Read the model definition and answer for the solid it produces. Units are mm, in the model's axes. A direction names the side the tool comes from. Coordinates: 2 decimals unless noted, no trailing zeros. Loops run counter-clockwise (first coordinate to the right, second up) from the corner with the lowest first, then second, coordinate; pieces in that order, holes last.
Q1. Straight lines are drawn through the part: line 1 (Y direction, x = 0, z = 95.7); line 2 (Z direction, x = 158, y = 115); line 3 (Y direction, x = 0, z = -96.3). For each, find the intervals that lie inside material, in ascending order.
Q2. Flat-ended cylindrical pins translate along their axes: P1, Ø2.5, axis at y = 77, z = 96.5, coming from the -X side (3 decimals); P2, Ø7, axis at x = -225.92, z = 85.26, coming from the -Y side. Find the tip coordinate at first contact, or state that the pin passes through.
Q3. Section A-A (y = 68.5) is taken. Give the vertices of the cut face in (x, z) (3 decimals).
Q4. Section C-C (z = 20.5) is taken. Give the vertices of the cut face in (x, y) (3 decimals), then the cut area to 3 significant figures.
Q5. Section B-B (x = 84) is taken. Give the vertices of the cut face in (y, z).
Q6. Which of the six approach directions +Z, -Z, +X, -X, +Y, -Y give full straight-line access (tool end or side, diameter ignored) to faces 1 (the face through (-3, 64, 95)), 2 (the face through (-3, -3.18, -1))?
Q7. The mould has two halves that part along Z. Classify faces 3 (the face through (-3, 0, -1)), 4 (the face through (-3, 64, -98.18)), 5 (the face through (-235.915, -0.4, 15)): pulls with the +Z half, pulls with the -Z half, needs draft (parallel to the pull), parting line crosses it, or undercut.
from build123d import *

# Parameters (mm, degrees)
BASE_FLANGE2_DEPTH      = 3.18
SKETCHED_START          = -235.915
SKETCHED_BEND1_DEPTH    = 471.83
SKETCHED_BEND1_2_DEPTH  = 471.83
CUT_EXTRUDE1_DEPTH      = 333.865793556
CUT_EXTRUDE1_DEPTH_BACK = 333.865793556
CUT_EXTRUDE2_DEPTH      = 333.865793556
CUT_EXTRUDE2_DEPTH_BACK = 333.865793556
SKETCH13_R              = 3
CUT_EXTRUDE3_DEPTH      = 288.595040156
CUT_EXTRUDE3_DEPTH_BACK = 288.595040156
SKETCH14_R              = 3


# Read off the part's stored shape, not the designer's step: Sketched Bend1
# Sheet-metal steps are written as plain solids
with BuildPart() as part:
    # Sketch1 → Base-Flange2 (new body)
    with BuildSketch(Plane(origin=(0, 0, 0), x_dir=(1, 0, 0), z_dir=(0, 1, 0))):
        Polygon((-235.915, -95), (-235.915, -225.97), (235.915, -225.97), (235.915, -95), (235.915, 95), (235.915, 225.97), (-235.915, 225.97), (-235.915, 95), align=None)
    extrude(amount=-BASE_FLANGE2_DEPTH)

    # Sketched Bend1 outline → Sketched Bend1 (cut)
    with BuildSketch(Plane.YZ.offset(SKETCHED_START)):
        with BuildLine():
            ThreePointArc((0, -98.110109763), (-2.282068839, -96.758874704), (-3.18, -94.2634))
            Line((-3.18, -94.2634), (-3.18, -225.97))
            Line((-3.18, -225.97), (0, -225.97))
            Line((0, -225.97), (0, -98.110109763))
        make_face()
        with BuildLine():
            Line((-3.18, 225.97), (-3.18, 94.2634))
            ThreePointArc((-3.18, 94.2634), (-2.282068839, 96.758874704), (0, 98.110109763))
            Line((0, 98.110109763), (0, 225.97))
            Line((0, 225.97), (-3.18, 225.97))
        make_face()
    extrude(amount=SKETCHED_BEND1_DEPTH, mode=Mode.SUBTRACT)

    # Sketched Bend1 2 outline → Sketched Bend1 2 (add)
    with BuildSketch(Plane.YZ.offset(SKETCHED_START)):
        with BuildLine():
            Line((0, -94.2634), (0, -98.110109763))
            ThreePointArc((0, -98.110109763), (0.366645879, -98.162488292), (0.7366, -98.18))
            Line((0.7366, -98.18), (128.788585266, -98.18))
            Line((128.788585266, -98.18), (128.788585266, -95))
            Line((128.788585266, -95), (0.7366, -95))
            ThreePointArc((0.7366, -95), (0.215745145, -94.784254855), (0, -94.2634))
        make_face()
        with BuildLine():
            ThreePointArc((0.7366, 98.18), (0.366645879, 98.162488292), (0, 98.110109763))
            Line((0, 98.110109763), (0, 94.2634))
            ThreePointArc((0, 94.2634), (0.215745145, 94.784254855), (0.7366, 95))
            Line((0.7366, 95), (128.788585266, 95))
            Line((128.788585266, 95), (128.788585266, 98.18))
            Line((128.788585266, 98.18), (0.7366, 98.18))
        make_face()
    extrude(amount=SKETCHED_BEND1_2_DEPTH)

    # Sketch11 → Cut-Extrude1 (cut, two sides: drawn at the far end of the back side and taken through both)
    with BuildSketch(Plane(origin=(0, 0, -98.18), x_dir=(-1, 0, 0), z_dir=(0, 0, -1)).offset(-CUT_EXTRUDE1_DEPTH_BACK)):
        with BuildLine():
            Line((-238.915, 18.3066), (-218.398065726, 18.3066))
            ThreePointArc((-218.398065726, 18.3066), (-215.338826457, 19.14510263), (-213.134647247, 21.426248301))
            Line((-213.134647247, 21.426248301), (-207.15158152, 32.359419665))
            ThreePointArc((-207.15158152, 32.359419665), (-206.602061377, 33.753250405), (-206.415, 35.239771364))
            Line((-206.415, 35.239771364), (-206.415, 95.705413902))
            ThreePointArc((-206.415, 95.705413902), (-206.602061377, 97.191934861), (-207.15158152, 98.585765601))
            Line((-207.15158152, 98.585765601), (-213.134647247, 109.518936965))
            ThreePointArc((-213.134647247, 109.518936965), (-215.338826457, 111.800082636), (-218.398065726, 112.638585266))
            Line((-218.398065726, 112.638585266), (-238.915, 112.638585266))
            Line((-238.915, 112.638585266), (-238.915, 18.3066))
        make_face()
        with BuildLine():
            Line((218.398065726, 112.638585266), (238.915, 112.638585266))
            Line((238.915, 112.638585266), (238.915, 18.3066))
            Line((238.915, 18.3066), (218.398065726, 18.3066))
            ThreePointArc((218.398065726, 18.3066), (215.338826457, 19.14510263), (213.134647247, 21.426248301))
            Line((213.134647247, 21.426248301), (207.15158152, 32.359419665))
            ThreePointArc((207.15158152, 32.359419665), (206.602061377, 33.753250405), (206.415, 35.239771364))
            Line((206.415, 35.239771364), (206.415, 95.705413902))
            ThreePointArc((206.415, 95.705413902), (206.602061377, 97.191934861), (207.15158152, 98.585765601))
            Line((207.15158152, 98.585765601), (213.134647247, 109.518936965))
            ThreePointArc((213.134647247, 109.518936965), (215.338826457, 111.800082636), (218.398065726, 112.638585266))
        make_face()
    extrude(amount=CUT_EXTRUDE1_DEPTH + CUT_EXTRUDE1_DEPTH_BACK, mode=Mode.SUBTRACT)

    # Sketch13 → Cut-Extrude2 (cut, two sides: drawn at the far end of the back side and taken through both)
    with BuildSketch(Plane(origin=(0, 0, -98.18), x_dir=(-1, 0, 0), z_dir=(0, 0, -1)).offset(-CUT_EXTRUDE2_DEPTH_BACK)):
        with Locations(Location((-195.915, 119.788585266, 0), (0, 0, 90))):
            Circle(SKETCH13_R)
        with Locations(Location((-195.915, 9.7366, 0), (0, 0, 90))):
            Circle(SKETCH13_R)
        with Locations(Location((195.915, 9.7366, 0), (0, 0, 90))):
            Circle(SKETCH13_R)
        with Locations(Location((195.915, 119.788585266, 0), (0, 0, 90))):
            Circle(SKETCH13_R)
        with Locations(Location((0, 119.788585266, 0), (0, 0, 90))):
            Circle(SKETCH13_R)
        with Locations(Location((0, 9.7366, 0), (0, 0, 90))):
            Circle(SKETCH13_R)
    extrude(amount=CUT_EXTRUDE2_DEPTH + CUT_EXTRUDE2_DEPTH_BACK, mode=Mode.SUBTRACT)

    # Sketch14 → Cut-Extrude3 (cut, two sides: drawn at the far end of the back side and taken through both)
    with BuildSketch(Plane.XZ.offset(3.18).offset(-CUT_EXTRUDE3_DEPTH_BACK)):
        with Locations(Location((-225.915, 85.2634, 0), (0, 0, 270))):
            Circle(SKETCH14_R)
        with Locations(Location((-225.915, -85.2634, 0), (0, 0, 270))):
            Circle(SKETCH14_R)
        with Locations(Location((225.915, -85.2634, 0), (0, 0, 270))):
            Circle(SKETCH14_R)
        with Locations(Location((225.915, 85.2634, 0), (0, 0, 270))):
            Circle(SKETCH14_R)
        with Locations(Location((0, 85.2634, 0), (0, 0, 270))):
            Circle(SKETCH14_R)
        with Locations(Location((0, -85.2634, 0), (0, 0, 270))):
            Circle(SKETCH14_R)
    extrude(amount=CUT_EXTRUDE3_DEPTH + CUT_EXTRUDE3_DEPTH_BACK, mode=Mode.SUBTRACT)


solid = part.part
Numbers:
1. line 1: y = -2.91 to 6.74, 12.74 to 116.79, 122.79 to 128.79
1. line 2: z = -98.18 to -95, 95 to 98.18
1. line 3: y = -2.61 to 6.74, 12.74 to 116.79, 122.79 to 128.79
2. P1: stops at x = -206.415
2. P2: stops at y = -3.18
3. outline: (-206.415, -98.18) - (206.415, -98.18) - (206.415, -95) - (-206.415, -95) - close; (-206.415, 95) - (206.415, 95) - (206.415, 98.18) - (-206.415, 98.18) - close
4. outline: (-235.915, -3.18) - (235.915, -3.18) - (235.915, 0) - (-235.915, 0) - close
4. area: 1,500 mm2
5. outline: (-3.18, -94.26) arc R3.92 ccw to (0.74, -98.18) - (128.79, -98.18) - (128.79, -95) - (0.74, -95) arc R0.74 cw to (0, -94.26) - (0, 94.26) arc R0.74 cw to (0.74, 95) - (128.79, 95) - (128.79, 98.18) - (0.74, 98.18) arc R3.92 ccw to (-3.18, 94.26) - close
6. face 1: +X, -X, +Y
6. face 2: +Z, -Z, +X, -X, -Y
7. face 3: undercut
7. face 4: pulls with the -Z half
7. face 5: needs draft
